The figure shows three views and two pictorial views of one solid part (mm, origin at its lowest corner). Answer the questions. A direction names the side the tool comes from. Round coordinates to 2 decimals unless told otherwise and drop trailing zeros. Write each loop counter-clockwise with the first axis right and the second up, starting at its lowest first coordinate (ties: lowest second). Pieces come first, ordered by that corner, then holes. Notation, with made-up numbers: M -17.5,0 L 35.5,0 A10 ccw 35.5,6 Z; hole C 17.5,-6 d9. An arc over 180 degrees is marked long. One line per item, written item: value. Start each with the question number.
Q1. Given pin 1 Ø12 at (x, y) = (30.5, 7.5) entering from +Z (1 decimal); pin 2 Ø5 at (x, y) = (13.5, 6) entering from -Z; pin 3 Ø19.5 at (x, z) = (23.93, 23.68) entering from +Y, each flat-ended and moving along its own axis, determine where each tip first touches the part or whether it passes through.
Q2. Find section B-B (z = 32). Write down the section's boundary in (x, y) (1 decimal).
Q3. A tool of negligible diameter and unlimited length cuts with its end or side. For the marked faces 1 and 2, from which of +Z, -Z, +X, -X, +Y, -Y can it reach the whole face along a straight path? Write none if from no direction.
Q4. Find section C-C (y = 30). Write down the section's boundary in (x, z) (1 decimal).
Q5. Consider probe 1 along X at (y, z) = (18, 23.5); probe 2 along X at (y, z) = (32, 33.5) (1 decimal); probe 3 along Y at (x, z) = (10, 2). Determine where each line is inside the solid, lowest interval first.
Q6. Find section D-D (x = 39.5). Write down the section's boundary in (y, z) (1 decimal), and give its area (3 significant figures).
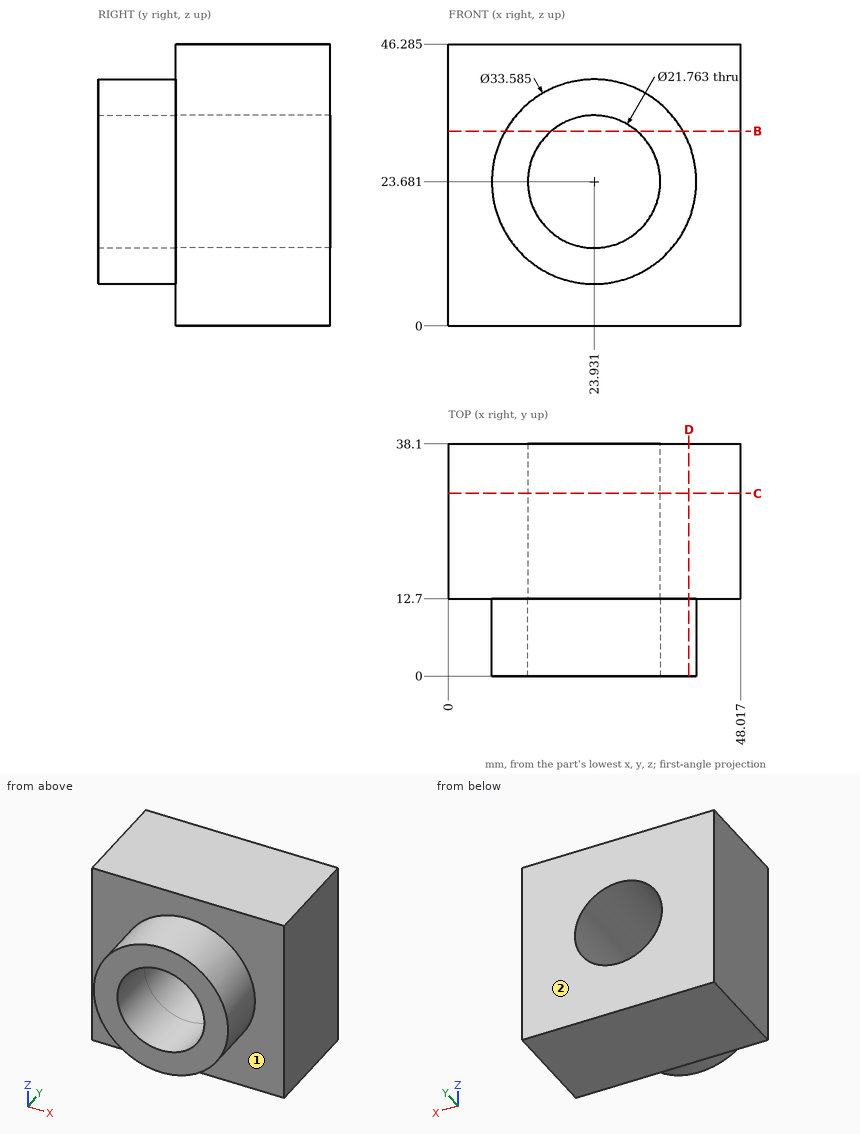
The answers:
1. pin 1: z = 46.3
1. pin 2: z = 8.88
1. pin 3: through
2. outline: M 0,12.7 L 9.3,12.7 L 9.3,0 L 16.9,0 L 16.9,38.1 L 0,38.1 Z; M 30.9,0 L 38.5,0 L 38.5,12.7 L 48,12.7 L 48,38.1 L 30.9,38.1 Z
3. face 1: -Y
3. face 2: +Z, -Z, +X, -X, +Y
4. outline: M 0,0 L 48,0 L 48,46.3 L 0,46.3 Z; hole C 23.9,23.7 d21.8
5. probe 1: 0 to 13.05, 34.81 to 48.02
5. probe 2: 0 to 19.2, 28.6 to 48
5. probe 3: 12.7 to 38.1
6. outline: M 0,17.4 L 12.7,17.4 L 12.7,0 L 38.1,0 L 38.1,46.3 L 12.7,46.3 L 12.7,30 L 0,30 Z
6. area: 1,340 mm2
